CAD build for the part. Positions are in the model's coordinates, mm. A direction names the side the tool comes from. Round coordinates to 2 decimals unless told otherwise and drop trailing zeros. Order: outer loops, then holes, each group sorted by start corner. A loop starts at its lowest first (then second) coordinate and runs counter-clockwise, first axis right, second up. Notation, with made-up numbers: M -23,-37 L 14,-37 A34 cw 14,2 Z; hole C -7.5,86.25 d7. An arc over 180 degrees is marked long. Put each result on its own line as item: value.
```python
from build123d import *

# Parameters (mm, degrees)
SKETCH001_W     = 9.016991
SKETCH001_H     = 9.88356
PAD_DEPTH       = 0.6
SKETCH002_W     = 4
SKETCH002_H     = 9.325613
POCKET_DEPTH    = 0.3
SKETCH003_W     = 4
SKETCH003_H     = 4
POCKET001_DEPTH = 0.3


with BuildPart() as part:
    # Sketch → Revolution (revolve)
    with BuildSketch(Plane.XY):
        Polygon((2, 7), (4, 7), (4, 12), (9, 12), (11, 0), (2, 0), align=None)
    revolve(axis=Axis((0, 0, 0), (0, 1, 0)))

    # Sketch001 (on Face1 of Revolution) → Pad (new body)
    with BuildSketch(Plane(origin=(0, 7, 0), x_dir=(-1, 0, 0), z_dir=(0, 1, 0))):
        with Locations((0.148778, -0.086759)):
            Rectangle(SKETCH001_W, SKETCH001_H)
    extrude(amount=PAD_DEPTH)

    # Sketch002 (on Face7 of Pad) → Pocket (cut)
    with BuildSketch(Plane(origin=(0, 7.6, 0), x_dir=(-1, 0, 0), z_dir=(0, 1, 0))):
        with Locations((0, -0.25022)):
            Rectangle(SKETCH002_W, SKETCH002_H)
    extrude(amount=-POCKET_DEPTH, mode=Mode.SUBTRACT)

    # Sketch003 (on Face3 of Pocket) → Pocket001 (cut)
    with BuildSketch(Plane.XZ.offset(-7)):
        Rectangle(SKETCH003_W, SKETCH003_H)
    extrude(amount=-POCKET001_DEPTH, mode=Mode.SUBTRACT)


solid = part.part
```
Item 1: Tool access for faces 5 (the flat face through (0, 7.3, 3)), 6 (the flat face through (-2, 12, 4)), 7 (the flat face through (-1.6, 7, -1.5)): list every direction of +Z, -Z, +X, -X, +Y, -Y with a clear straight run to the whole face (end or side of a thin tool).
Answers below:
face 5: none
face 6: +Z, -Z, +X, -X, +Y
face 7: +Y
Item 2: Pin check, flat tips, straight feed: P1, Ø2.5, axis at x = -0.5, z = 3, coming from the +Y side; P2, Ø1, axis at x = 3, z = 1.5, coming from the +Y side; P3, Ø1.6, axis at x = -1, z = -1, coming from the +Y side; P4, Ø1, axis at x = 5.5, y = 9, coming from the -Z side. Stop position of each tip, or through.
Answers below:
P1: y = 12
P2: y = 7.6
P3: y = 7
P4: z = -8.09
Item 3: Band-saw the part on A-A on y = 9. Give the cut face in (x, z).
Answers below:
outline: C 0,0 d19; hole C 0,0 d8
Item 4: Probe line 1 along Z through (x, y) = (0, 10.5); line 2 along X through (y, z) = (10.8, 0); line 3 along Y through (x, z) = (0, -3.5). List the from-to ranges inside material, lowest first. Write a range as [from, to].
Answers below:
line 1: [-9.25, -4], [4, 9.25]
line 2: [-9.2, -4], [4, 9.2]
line 3: [0, 7.3]
Item 5: Band-saw the part on B-B on y = 5.25. Give the cut face in (x, z) (3 decimals).
Answers below:
outline: C 0,0 d20.25; hole C 0,0 d4
Item 6: Mould opens along Y. For faces 1 (the cylindrical face through (0, 4, 2)), 2 (the flat face through (-0.2, 0, 2.3)), 3 (the flat face through (0, 7.3, -3)), 4 (the flat face through (-1.6, 7, 1.5)) say: pulls with the +Y half, pulls with the -Y half, needs draft (parallel to the pull), parting line crosses it, or undercut.
Answers below:
face 1: needs draft
face 2: pulls with the -Y half
face 3: undercut
face 4: pulls with the +Y half
